```python
from build123d import *

# Parameters (mm, degrees)
BOSS_EXTRUDE1_DEPTH = 2
SKETCH2_W           = 7
SKETCH2_H           = 1.45
BOSS_EXTRUDE2_DEPTH = 3
SKETCH3_W           = 6.349281592
SKETCH3_H           = 1
BOSS_EXTRUDE3_DEPTH = 2


with BuildPart() as part:
    # Sketch1 → Boss-Extrude1 (new body)
    with BuildSketch(Plane(origin=(0, 0, 0), x_dir=(1, 0, 0), z_dir=(0, 1, 0))):
        Polygon((12.5, -4.5), (21.5, -4.5), (21.5, 19.5), (12.5, 19.5), (12.5, 4.5), (-12.5, 4.5), (-12.5, 6), (-19.5, 6), (-19.5, -6), (-12.5, -6), (-12.5, -4.5), align=None)
    extrude(amount=BOSS_EXTRUDE1_DEPTH)

    # Sketch2 → Boss-Extrude2 (add)
    with BuildSketch(Plane(origin=(0, 0, 0), x_dir=(1, 0, 0), z_dir=(0, 1, 0))):
        Polygon((-13.150718408, 4.5), (12.5, 4.5), (12.5, 19.5), (14, 19.5), (14, 3), (-13.150718408, 3), align=None)
        Polygon((20, 19.5), (20, -3), (-13.150718408, -3), (-13.150718408, -4.5), (21.5, -4.5), (21.5, 19.5), align=None)
        Polygon((-13.150718408, 1), (16, 1), (16, 19.5), (18, 19.5), (18, -1), (-13.150718408, -1), align=None)
        with Locations((-16, 5.275)):
            Rectangle(SKETCH2_W, SKETCH2_H)
        with Locations((-16, -5.275)):
            Rectangle(SKETCH2_W, SKETCH2_H)
    extrude(amount=-BOSS_EXTRUDE2_DEPTH)

    # Sketch3 → Boss-Extrude3 (add)
    with BuildSketch(Plane.XZ.offset(3)):
        with Locations((-16.325359204, 4.05)):
            Rectangle(SKETCH3_W, SKETCH3_H)
        with Locations((-16.325359204, -4.05)):
            Rectangle(SKETCH3_W, SKETCH3_H)
    extrude(amount=-BOSS_EXTRUDE3_DEPTH)


solid = part.part
```
Input: part model. Units: mm. Frame: model coordinates. A direction names the side the tool comes from. Give positions to 0.01 mm unless a question says otherwise; leave off trailing zeros. Order: outer loops, then holes, each group sorted by start corner. A loop starts at its lowest first (then second) coordinate and runs counter-clockwise, first axis right, second up. Notation, with made-up numbers: M 18,48.5 L 61,48.5 A33 cw 61,83.5 Z; hole C 78,-4.75 d8. An arc over 180 degrees is marked long. Return JSON: item names as keys, results as strings.
Item 1: Ray query, probe 1 along Z at (x, y) = (-4, -0.8); probe 2 along X at (y, z) = (-1.35, -5.5); probe 3 along X at (y, z) = (-0.15, -7.5). Return the intervals inside material, ascending.
Solutions:
{"probe 1": "-4.5 to -3, -1 to 1, 3 to 4.5", "probe 2": "-19.5 to -12.5, 12.5 to 14, 16 to 18, 20 to 21.5", "probe 3": "12.5 to 14, 16 to 18, 20 to 21.5"}
Item 2: Cut plane B-B (z = -8.5). Return loops of the section in (x, y).
Solutions:
{"outline": "M 12.5,-3 L 14,-3 L 14,0 L 16,0 L 16,-3 L 18,-3 L 18,0 L 20,0 L 20,-3 L 21.5,-3 L 21.5,2 L 12.5,2 Z"}
Item 3: Cut plane A-A (y = -2.35). State how many separate pieces and enclosed holes the cut face has, then the cut area to 3 significant figures.
Solutions:
{"separate pieces": "3", "enclosed holes": "0", "area": "281 mm^2"}
Item 4: Pull-direction query (X, two-part tool) for faces 1 (the flat face through (-16, -1, 6)), 2 (the flat face through (-12.5, -1, 5)), 3 (the flat face through (-1, 0, -4.5)); classes: +X half, -X half, draft (parallel to the pull), parting line (faces both ways), or undercut.
Solutions:
{"face 1": "draft", "face 2": "+X half", "face 3": "undercut"}
Item 5: Cut plane C-C (x = -6). Return loops of the section in (y, z).
Solutions:
{"outline": "M -3,-4.5 L 2,-4.5 L 2,4.5 L -3,4.5 L -3,3 L 0,3 L 0,1 L -3,1 L -3,-1 L 0,-1 L 0,-3 L -3,-3 Z"}
Item 6: Access query for faces 4 (the flat face through (8, -3, 0)), 5 (the flat face through (1, -1, -3)), 6 (the flat face through (-16, -1, 4)), 7 (the flat face through (-12.5, -1, -5)), 8 (the flat face through (18, -1, -9)). Directions: +Z, -Z, +X, -X, +Y, -Y. A direction counts if a zero-diameter tool reaches every point of the face in a straight line with its end or side. Return the directions, or none.
Solutions:
{"face 4": "+Z, -Z, +X, -X, -Y", "face 5": "-X, -Y", "face 6": "-X", "face 7": "-Z, +Y, -Y", "face 8": "-Z, -Y"}
Item 7: First-contact query: P1, Ø1.6, axis at y = -1.5, z = -0.5, coming from the -X side; P2, Ø1.5, axis at x = -2.5, y = -2, coming from the +Z side; P3, Ø1.5, axis at x = -16, y = -0.5, coming from the -Z side. Flat tips, straight axial feed; report the tip coordinate or a pass-through.
Solutions:
{"P1": "x = -13.15", "P2": "z = 4.5", "P3": "z = -6"}
Item 8: Cut plane D-D (y = 1.4). Return loops of the section in (x, z), then the cut area to 3 significant figures.
Solutions:
{"outline": "M -19.5,-6 L -12.5,-6 L -12.5,-4.5 L 12.5,-4.5 L 12.5,-19.5 L 21.5,-19.5 L 21.5,4.5 L -12.5,4.5 L -12.5,6 L -19.5,6 Z", "area": "525 mm^2"}
